```python
from build123d import *

# Parameters (mm, degrees)
F0_W     = 150
F0_H     = 150
F1_DEPTH = 3
F2_W     = 3
F2_H     = 7
F3_DEPTH = 150
F2_R     = 10
F2_W_2   = 27
F2_H_2   = 1.5
F4_DEPTH = 3.001


with BuildPart() as f1:
    # F0 (on Front) → F1 (new body)
    with BuildSketch(Plane.XZ):
        Rectangle(F0_W, F0_H)
    extrude(amount=F1_DEPTH)

    # F2 (on face) → F3 (join)
    with BuildSketch(Plane.XZ.offset(3)):
        Polygon((-36.712797, 15), (-30.754029, 20), (-32.682392, 22.298133), (-39.712797, 16.398923), (-39.712797, -16.091911), (-31.398923, -26), (31.398923, -26), (39.712797, -16.091911), (39.712797, 16.091911), (34.815432, 21.928363), (32.517299, 20), (36.712797, 15), (36.712797, -15), (30, -23), (22, -23), (19, -23), (-19, -23), (-22, -23), (-30, -23), (-36.712797, -15), align=None)
        with Locations((-20.5, -19.5)):
            Rectangle(F2_W, F2_H)
        Polygon((-31.5, -12.9), (-34.07115, -9.835822), (-36.369284, -11.764185), (-32.898923, -15.9), (32.898923, -15.9), (36.369284, -11.764185), (34.07115, -9.835822), (31.5, -12.9), align=None)
        with Locations((20.5, -19.5)):
            Rectangle(F2_W, F2_H)
    extrude(amount=F3_DEPTH)

    # F2 (on face) → F4 (cut, through all)
    with BuildSketch(Plane.XZ.offset(3)):
        with Locations((0, 12)):
            Circle(F2_R)
        with BuildLine():
            ThreePointArc((-29, -17), (-29.707107, -17.292893), (-30, -18))
            Line((-30, -18), (-30, -21))
            ThreePointArc((-30, -21), (-29.707107, -21.707107), (-29, -22))
            Line((-29, -22), (-24, -22))
            ThreePointArc((-24, -22), (-23.292893, -21.707107), (-23, -21))
            Line((-23, -21), (-23, -18))
            ThreePointArc((-23, -18), (-23.292893, -17.292893), (-24, -17))
            Line((-24, -17), (-29, -17))
        make_face()
        with BuildLine():
            Line((17, -17), (-17, -17))
            ThreePointArc((-17, -17), (-17.707107, -17.292893), (-18, -18))
            Line((-18, -18), (-18, -21))
            ThreePointArc((-18, -21), (-17.707107, -21.707107), (-17, -22))
            Line((-17, -22), (17, -22))
            ThreePointArc((17, -22), (17.707107, -21.707107), (18, -21))
            Line((18, -21), (18, -18))
            ThreePointArc((18, -18), (17.707107, -17.292893), (17, -17))
        make_face()
        with BuildLine():
            Line((29, -17), (24, -17))
            ThreePointArc((24, -17), (23.292893, -17.292893), (23, -18))
            Line((23, -18), (23, -21))
            ThreePointArc((23, -21), (23.292893, -21.707107), (24, -22))
            Line((24, -22), (29, -22))
            ThreePointArc((29, -22), (29.707107, -21.707107), (30, -21))
            Line((30, -21), (30, -18))
            ThreePointArc((30, -18), (29.707107, -17.292893), (29, -17))
        make_face()
        with BuildLine():
            Line((2.5, -4.9), (-2.5, -4.9))
            ThreePointArc((-2.5, -4.9), (-3.207107, -5.192893), (-3.5, -5.9))
            Line((-3.5, -5.9), (-3.5, -10.9))
            ThreePointArc((-3.5, -10.9), (-3.207107, -11.607107), (-2.5, -11.9))
            Line((-2.5, -11.9), (2.5, -11.9))
            ThreePointArc((2.5, -11.9), (3.207107, -11.607107), (3.5, -10.9))
            Line((3.5, -10.9), (3.5, -5.9))
            ThreePointArc((3.5, -5.9), (3.207107, -5.192893), (2.5, -4.9))
        make_face()
        with Locations((-19, -7.35)):
            Rectangle(F2_W_2, F2_H_2)
        with Locations((-19, -9.85)):
            Rectangle(F2_W_2, F2_H_2)
        with Locations((19, -7.35)):
            Rectangle(F2_W_2, F2_H_2)
        with Locations((19, -9.85)):
            Rectangle(F2_W_2, F2_H_2)
    extrude(amount=-F4_DEPTH, mode=Mode.SUBTRACT)


solid = f1.part
```
CAD build for the part. Positions are in the model's coordinates, mm. A direction names the side the tool comes from. Coordinates: 2 decimals unless noted, no trailing zeros. Order: outer loops, then holes, each group sorted by start corner. A loop starts at its lowest first (then second) coordinate and runs counter-clockwise, first axis right, second up. Notation, with made-up numbers: (65.5, 89) -> (86.5, 89) arc R18 ccw to (86.5, 96) -> close; hole circle Ø9 at (20, -37.75). An arc over 180 degrees is marked (long way). Use one line per item in the form item = value. Start each with the question number.
1) Drop flat-ended pins along their axis: pin 1 (2.5 mm diameter, centred on x = 20.5, y = -49, fed in from +Z); pin 2 (3.5 mm diameter, centred on y = -89, z = -18, fed in from +X); pin 3 (6 mm diameter, centred on x = -40.5, y = -37, fed in from -Z); pin 4 (10 mm diameter, centred on y = -106.5, z = -34, fed in from +X). Give the stop position or say it passes through.
2) Drill centre lines: L1, parallel to Z at x = 0, y = -1.4; L2, parallel to X at y = -117, z = 2.5; L3, parallel to Z at x = 33.5, y = -106. Where is each one in solid material? Low to high. Write a range as [from, to].
3) Tool access for faces 5 (the cylindrical face through (-2.17, -1.52, 2.24)), 6 (the flat face through (37.3, -76.95, 18.97)), 7 (the flat face through (34.586, -76.95, 17.535)), 8 (the flat face through (35.498, -76.95, -21.115)): list every direction of +Z, -Z, +X, -X, +Y, -Y with a clear straight run to the whole face (end or side of a thin tool).
4) Band-saw the part on C-C on z = 12. Give the cut face in (x, y).
5) Band-saw the part on D-D on z = -34. Give the cut face in (x, y), then the cut area to 3 significant figures.
6) Band-saw the part on B-B on x = 0. Give the cut face in (y, z), then the cut area to 3 significant figures.
7) Pull direction Z, two halves, no side cores. Call faces 1 (the flat face through (2.8, -153, -23.2)), 2 (the flat face through (-22, -77, -20)), 3 (the flat face through (-36.15, -76.95, 19.39)), 4 (the flat face through (19, -77, -20)): +Z half, -Z half, draft (parallel to the pull), parting line (faces both ways), or undercut.
Entries:
q1.pin_1 = -12.9
q1.pin_2 = 39.58
q1.pin_3 = -18.73
q1.pin_4 = through
q2.L1 = [-75, -22], [-17, -11.9], [-4.9, 2], [22, 75]
q2.L2 = [-39.71, -36.71], [36.71, 39.71]
q2.L3 = [-23.5, -18.83], [-15.18, -10.52], [18.83, 20.82]
q3.face_5 = +Y, -Y
q3.face_6 = +Z, +X, -Y
q3.face_7 = -Y
q3.face_8 = -Z, +X, -Y
q4.outline = (-75, -3) -> (-39.71, -3) -> (-39.71, -153) -> (-36.71, -153) -> (-36.71, -3) -> (-10, -3) -> (-10, 0) -> (-75, 0) -> close; (10, -3) -> (36.71, -3) -> (36.71, -153) -> (39.71, -153) -> (39.71, -3) -> (75, -3) -> (75, 0) -> (10, 0) -> close
q5.outline = (-75, -3) -> (75, -3) -> (75, 0) -> (-75, 0) -> close
q5.area = 450 mm2
q6.outline = (-153, -26) -> (-3, -26) -> (-3, -75) -> (0, -75) -> (0, -22) -> (-3, -22) -> (-3, -23) -> (-153, -23) -> close; (-153, -15.9) -> (-3, -15.9) -> (-3, -17) -> (0, -17) -> (0, -11.9) -> (-3, -11.9) -> (-3, -12.9) -> (-153, -12.9) -> close; (-3, -4.9) -> (0, -4.9) -> (0, 2) -> (-3, 2) -> close; (-3, 22) -> (0, 22) -> (0, 75) -> (-3, 75) -> close
q6.area = 1,250 mm2
q7.face_1 = draft
q7.face_2 = undercut
q7.face_3 = +Z half
q7.face_4 = undercut
